```python
from build123d import *

# Parameters (mm, degrees)
BOX_W     = 10
BOX_H     = 17
BOX_DEPTH = 50
PAD_DEPTH = 50
FILLET_R  = 2


with BuildPart() as cube:
    # Box → Box (new body)
    with BuildSketch(Plane(origin=(40, 0, 0), x_dir=(1, 0, 0), z_dir=(0, 0, 1))):
        with Locations((5, 8.5)):
            Rectangle(BOX_W, BOX_H)
    extrude(amount=BOX_DEPTH)


with BuildPart() as fillet_body:
    # Sketch → Pad (new body)
    with BuildSketch(Plane.XY):
        Polygon((0, 0), (0, 83), (5, 83), (5, 23), (113, 23), (113, 83), (118, 83), (118, 13), (47.289322, -57.710678), (41.959322, -52.380678), (107.34, 13), (5, 13), (5, 0), align=None)
    extrude(amount=PAD_DEPTH)

    # Fusion: union Cube
    add(cube.part)

    # Fillet
    fillet_edges = [fillet_body.edges().sort_by_distance(p)[0] for p in [
        (0, 0, 25),
        (0, 83, 25),
        (5, 0, 25),
        (5, 83, 25),
        (5, 13, 25),
        (5, 23, 25),
        (113, 23, 25),
        (113, 83, 25),
        (118, 83, 25),
        (47.289322, -57.710678, 25),
        (41.959322, -52.380678, 25),
        (107.34, 13, 25),
        (50, 13, 25),
        (40, 13, 25),
        (50, 0, 25),
        (40, 0, 25),
    ]]
    fillet(fillet_edges, radius=FILLET_R)


solid = fillet_body.part
```
Could you check a few things on this model? Use its own coordinates, in mm. A direction names the side the tool comes from. Round coordinates to 2 decimals unless told otherwise and drop trailing zeros. Loops run counter-clockwise (first coordinate to the right, second up) from the corner with the lowest first, then second, coordinate; pieces in that order, holes last.
Q1. On a 3-axis mill with a long thin cutter (end or side, diameter ignored), from which of +Z, -Z, +X, -X, +Y, -Y can I reach the whole of each face in a straight line? I mean faces 1 (the flat face through (58, 23, 25)), 2 (the flat face through (5, 7, 25)), 3 (the flat face through (63.1, 13.4, 50)), 4 (the flat face through (45, 0, 25)), 5 (the flat face through (50, 6, 25)). Say none if no direction works.
Q2. I want a section at A-A (y = 52). Write out the boundary of the cut face in (x, z).
Q3. I want a section at B-B (y = 7). Write out the boundary of the cut face in (x, z), and give its area (3 significant figures).
Q4. For P1, Ø1, axis at x = 37, z = 13.5, coming from the -Y side; P2, Ø3, axis at x = 93.5, z = 23, coming from the +Y side; P3, Ø10, axis at y = -26.5, z = 30.5, coming from the +X side, each with a flat end and sliding along its axis, tell me the tip position at first contact or that it passes through.
Q5. Thinking about a two-plate mould opening in X: for faces 6 (the flat face through (0, 41, 25)), 7 (the flat face through (84, -21, 25)), 8 (the flat face through (78, 13, 25)), which applies, pulls with the +X half, pulls with the -X half, needs draft (parallel to the pull), parting line crosses it, or undercut?
Q6. Please list where these lines run through material, in increasing order: L1, parallel to X at y = 10.5, z = 9.5; L2, parallel to X at y = 12, z = 39; L3, parallel to X at y = 40.5, z = 19.
Q7. I want a section at C-C (x = 62.5). Write out the boundary of the cut face in (y, z).
Answer below:
1. face 1: +Z, -Z, +Y
1. face 2: +Z, -Z, -Y
1. face 3: +Z, +X, -X, +Y, -Y
1. face 4: +Z, -Z, -X
1. face 5: +Z, -Z
2. outline: (0, 0) - (5, 0) - (5, 50) - (0, 50) - close; (113, 0) - (118, 0) - (118, 50) - (113, 50) - close
3. outline: (0, 0) - (5, 0) - (5, 50) - (0, 50) - close; (40, 0) - (50, 0) - (50, 50) - (40, 50) - close; (101.34, 0) - (112, 0) - (112, 50) - (101.34, 50) - close
3. area: 1,280 mm2
4. P1: stops at y = 13
4. P2: stops at y = 23
4. P3: stops at x = 83.5
5. face 6: pulls with the -X half
5. face 7: pulls with the +X half
5. face 8: undercut
6. L1: x = 0 to 5, 40 to 50, 104.45 to 115.5
6. L2: x = 0 to 5.27, 39.73 to 50.27, 104.24 to 117
6. L3: x = 0 to 5, 113 to 118
7. outline: (-42.5, 0) - (-31.84, 0) - (-31.84, 50) - (-42.5, 50) - close; (13, 0) - (23, 0) - (23, 50) - (13, 50) - close
